Here's how the part is built. I have some questions about the finished solid (model axes, mm). A direction names the side the tool comes from. Round coordinates to 2 decimals unless told otherwise and drop trailing zeros. Order: outer loops, then holes, each group sorted by start corner. A loop starts at its lowest first (then second) coordinate and runs counter-clockwise, first axis right, second up. Notation, with made-up numbers: (7.5, 56.5) - (36.5, 56.5) arc R21 cw to (36.5, 93.5) - close; hole circle Ø6 at (56, 82.25). An arc over 180 degrees is marked (long way). Answer as a JSON object with one key per item and string values.
```python
from build123d import *

# Parameters (mm, degrees)
PAD_DEPTH       = 3
PAD001_DEPTH    = 3
SKETCH002_W     = 209.08447
SKETCH002_H     = 4.18
PAD002_DEPTH    = 3
SKETCH003_W     = 26.3
SKETCH003_H     = 34.2
POCKET_DEPTH    = 3
SKETCH004_W     = 18
SKETCH004_H     = 25
POCKET001_DEPTH = 3
SKETCH005_W     = 14
SKETCH005_H     = 5
POCKET002_DEPTH = 6
SKETCH006_W     = 14
SKETCH006_H     = 3
POCKET003_DEPTH = 3
SKETCH007_W     = 8
SKETCH007_H     = 3
POCKET004_DEPTH = 3
SKETCH008_W     = 200
SKETCH008_H     = 4.4
PAD003_DEPTH    = 3
SKETCH009_R     = 0.8
POCKET005_DEPTH = 9


with BuildPart() as part:
    # Sketch → Pad (new body)
    with BuildSketch(Plane.XY):
        with BuildLine():
            ThreePointArc((-100, 50), (-150, 0), (-100, -50))
            Line((-100, -50), (100, -50))
            ThreePointArc((100, -50), (150, 0), (100, 50))
            Line((-100, 50), (100, 50))
        make_face()
    extrude(amount=PAD_DEPTH)

    # Sketch001 (on Face6 of Pad) → Pad001 (join)
    with BuildSketch(Plane.XY.offset(3)):
        with BuildLine():
            ThreePointArc((-100, 50), (-150, 0), (-100, -50))
            Line((-100, -50), (100, -50))
            ThreePointArc((100, -50), (150, 0), (100, 50))
            Line((-100, 50), (100, 50))
        make_face()
        with BuildLine():
            ThreePointArc((-100, 5), (-105, 0), (-100, -5))
            Line((-100, -5), (100, -5))
            ThreePointArc((100, -5), (105, 0), (100, 5))
            Line((-100, 5), (100, 5))
        make_face(mode=Mode.SUBTRACT)
    extrude(amount=PAD001_DEPTH)

    # Sketch002 (on Face9 of Pad001) → Pad002 (join)
    with BuildSketch(Plane.XY.offset(6)):
        with BuildLine():
            ThreePointArc((-100, 50), (-150, 0), (-100, -50))
            Line((-100, -50), (100, -50))
            ThreePointArc((100, -50), (150, 0), (100, 50))
            Line((-100, 50), (100, 50))
        make_face()
        Rectangle(SKETCH002_W, SKETCH002_H, mode=Mode.SUBTRACT)
    extrude(amount=PAD002_DEPTH)

    # Sketch003 (on Face13 of Pad002) → Pocket (cut)
    with BuildSketch(Plane.XY.offset(9)):
        with Locations((0, -29.9)):
            Rectangle(SKETCH003_W, SKETCH003_H)
    extrude(amount=-POCKET_DEPTH, mode=Mode.SUBTRACT)

    # Sketch004 (on Face27 of Pocket) → Pocket001 (cut)
    with BuildSketch(Plane.XY.offset(6)):
        with Locations((0, -25.3)):
            Rectangle(SKETCH004_W, SKETCH004_H)
    extrude(amount=-POCKET001_DEPTH, mode=Mode.SUBTRACT)

    # Sketch005 (on Face13 of Pocket001) → Pocket002 (cut)
    with BuildSketch(Plane.XY.offset(9)):
        with Locations((0, -10.3)):
            Rectangle(SKETCH005_W, SKETCH005_H)
    extrude(amount=-POCKET002_DEPTH, mode=Mode.SUBTRACT)

    # Sketch006 (on Face23 of Pocket002) → Pocket003 (cut)
    with BuildSketch(Plane.XZ.offset(7.8)):
        with Locations((0, 4.5)):
            Rectangle(SKETCH006_W, SKETCH006_H)
    extrude(amount=-POCKET003_DEPTH, mode=Mode.SUBTRACT)

    # Sketch007 (on Face13 of Pocket003) → Pocket004 (cut)
    with BuildSketch(Plane.XY.offset(9)):
        with Locations((0, -48.5)):
            Rectangle(SKETCH007_W, SKETCH007_H)
    extrude(amount=-POCKET004_DEPTH, mode=Mode.SUBTRACT)

    # Sketch008 (on Face15 of Pocket004) → Pad003 (join)
    with BuildSketch(Plane.XY.offset(9)):
        with BuildLine():
            ThreePointArc((-100, 50), (-150, 0), (-100, -50))
            Line((-100, -50), (100, -50))
            ThreePointArc((100, -50), (150, 0), (100, 50))
            Line((-100, 50), (100, 50))
        make_face()
        Rectangle(SKETCH008_W, SKETCH008_H, mode=Mode.SUBTRACT)
    extrude(amount=PAD003_DEPTH)

    # Sketch009 (on Face4 of Pad003) → Pocket005 (cut)
    with BuildSketch(Plane(origin=(0, 0, 0), x_dir=(1, 0, 0), z_dir=(0, 0, -1))):
        with Locations((-95, 35)):
            Circle(SKETCH009_R)
        with Locations((-95, -35)):
            Circle(SKETCH009_R)
    pocket005 = extrude(amount=-POCKET005_DEPTH, mode=Mode.SUBTRACT)

    # Mirrored: Pocket005 across Sketch009 V_Axis
    add(pocket005.mirror(Plane(origin=(0, 0, 0), x_dir=(0, 0, -1), z_dir=(1, 0, 0))), mode=Mode.SUBTRACT)


solid = part.part
```
1. Imagine slicing it at B-B (x = -117). List the corners of the cut face in (y, z) for me.
Responses:
{"outline": "(-47.02, 0) - (47.02, 0) - (47.02, 12) - (-47.02, 12) - close"}
2. For P1, Ø3.5, axis at y = -0.5, z = 8, coming from the +X side; P2, Ø6, axis at y = -37.5, z = 6, coming from the +X side; P3, Ø0.9, axis at y = -36.5, z = 7.5, coming from the -X side, each with a flat end and sliding along its axis, tell me the tip position at first contact or that it passes through.
Responses:
{"P1": "x = 150", "P2": "x = 136.19", "P3": "x = -134.65"}
3. If I drill on L1, parallel to Y at x = -95, z = 4.5; L2, parallel to Y at x = 95, z = 6.75; L3, parallel to Y at x = 95, z = 2, over which ranges is the centre line in solid material (lowest first)? Write a range as [from, to].
Responses:
{"L1": "[-50, -35.8], [-34.2, -5], [5, 34.2], [35.8, 50]", "L2": "[-50, -35.8], [-34.2, -2.09], [2.09, 34.2], [35.8, 50]", "L3": "[-50, -35.8], [-34.2, 34.2], [35.8, 50]"}
4. Thinking about a two-plate mould opening in Y: for faces 3 (the face through (-1, 50, 6)), 4 (the face through (9, -12.8, 7)), 5 (the face through (149.988, -1.099, 5.916)), which applies, pulls with the +Y half, pulls with the -Y half, needs draft (parallel to the pull), parting line crosses it, or undercut?
Responses:
{"face 3": "pulls with the +Y half", "face 4": "undercut", "face 5": "parting line crosses it"}
5. For faces 1 (the face through (-149.988, 1.099, 5.916)), 2 (the face through (-9, -12.8, 7)), which set-ups out of +Z, -Z, +X, -X, +Y, -Y let a thin tool reach every point of the face, with its end or its side?
Responses:
{"face 1": "+Z, -Z, -X", "face 2": "none"}
6. Imagine slicing it at A-A (x = 20). List the corners of the cut face in (y, z) for me.
Responses:
{"outline": "(-50, 0) - (50, 0) - (50, 12) - (2.2, 12) - (2.2, 9) - (2.09, 9) - (2.09, 6) - (5, 6) - (5, 3) - (-5, 3) - (-5, 6) - (-2.09, 6) - (-2.09, 9) - (-2.2, 9) - (-2.2, 12) - (-50, 12) - close"}
